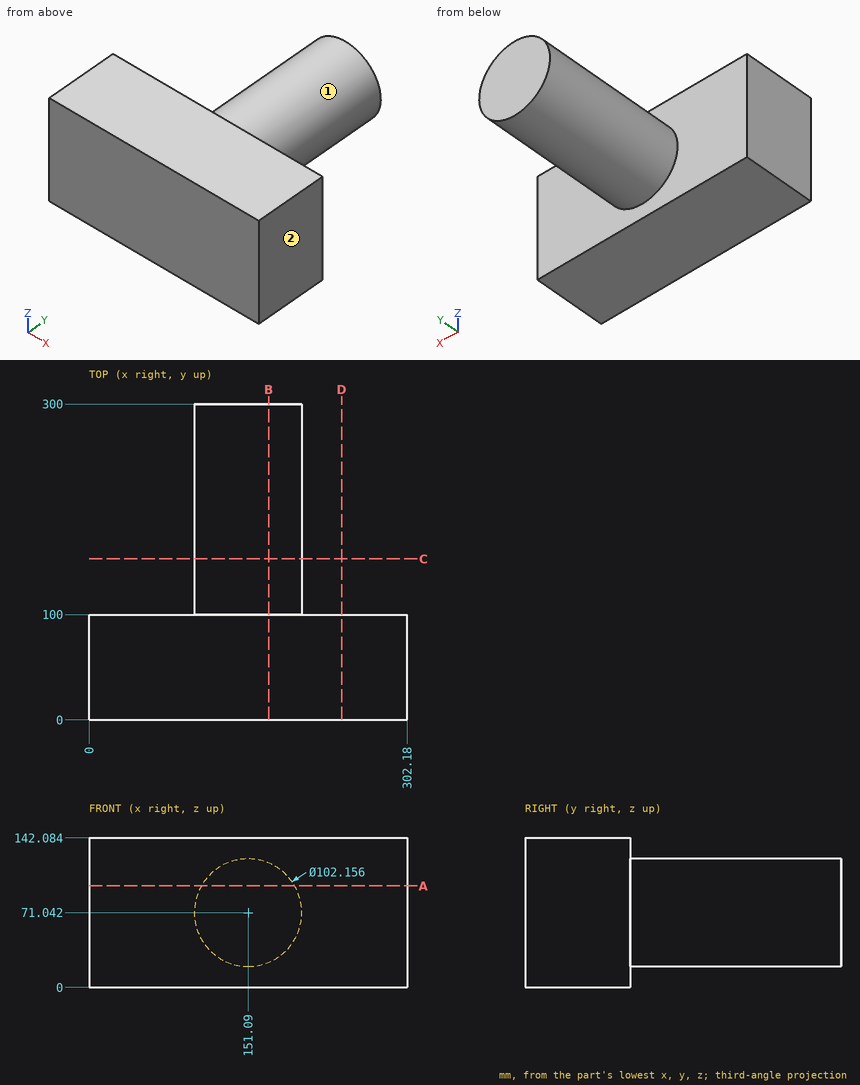
The drawing under review shows one solid part. Ordinate dimensions are in mm from its lowest x, y, z. A direction names the side the tool comes from. Coordinates: 2 decimals unless noted, no trailing zeros. Loops run counter-clockwise (first coordinate to the right, second up) from the corner with the lowest first, then second, coordinate; pieces in that order, holes last. Notation, with made-up numbers: M -6.5,15.25 L 14.5,15.25 A33 cw 14.5,52.25 Z; hole C 12,-5 d1. An arc over 180 degrees is marked long. Use one line per item in the form item = value.
(1) Clearance check with flat-ended pins moving along their axes: P1, Ø2, axis at y = 143, z = 38, coming from the -X side; P2, Ø6, axis at x = 170, y = 172.5, coming from the -Z side (1 decimal); P3, Ø12, axis at y = 188, z = 42.5, coming from the +X side (1 decimal). State where each tip first meets the part, or that it passes through.
Return value:
P1 = 111.31
P2 = 22.5
P3 = 196.9
(2) Consider section C-C (y = 153). Write out the cut boundary in (x, z).
Return value:
outline = C 151.09,71.04 d102.16
(3) Consider section B-B (x = 170.5). Write out the cut boundary in (y, z) (1 decimal), and give its area (3 significant figures).
Return value:
outline = M 0,0 L 100,0 L 100,23.8 L 300,23.8 L 300,118.3 L 100,118.3 L 100,142.1 L 0,142.1 Z
area = 33,100 mm2
(4) Consider section A-A (z = 96.5). Write out the cut boundary in (x, y), and give its area (3 significant figures).
Return value:
outline = M 0,0 L 302.18,0 L 302.18,100 L 195.37,100 L 195.37,300 L 106.81,300 L 106.81,100 L 0,100 Z
area = 47,900 mm2
(5) For line 1 along Y through (x, z) = (277.5, 35.5); line 2 along Z through (x, y) = (150, 108) (1 decimal); line 3 along X through (y, z) = (243, 115.5) (1 decimal), list the stretches that pass through material, from the lowest coordinate up. Write a range as from..to.
Return value:
line_1 = 0..100
line_2 = 20..122.1
line_3 = 125.9..176.2
(6) For the marked faces 1 and 2, list the 3-axis set-ups (+Z, -Z, +X, -X, +Y, -Y) from which the entire face can be reached by the end or side of a thin tool; tool diameter is ignored.
Return value:
face_1 = +Y
face_2 = +Z, -Z, +X, +Y, -Y
(7) Consider section D-D (x = 240). Write out the cut boundary in (y, z), and give its area (3 significant figures).
Return value:
outline = M 0,0 L 100,0 L 100,142.08 L 0,142.08 Z
area = 14,200 mm2
